Here's how the part is built. I have some questions about the finished solid (model axes, mm). Face numbers are marked on the shaded views. Coordinates: 2 decimals unless noted, no trailing zeros. Write each loop counter-clockwise with the first axis right and the second up, starting at its lowest first coordinate (ties: lowest second). Pieces come first, ordered by that corner, then holes.
Item 1: If I drill on line 1 (Z direction, x = 0, y = -9.75); line 2 (Z direction, x = 3, y = -16); line 3 (X direction, y = -3.5, z = -10), over which ranges is the centre line in solid material (lowest first)?
Item 2: I'm going to push flat-ended pins straight in: pin 1 Ø10 at (x, z) = (19, -15) entering from -Y; pin 2 Ø4 at (x, y) = (-11, -15.5) entering from +Z; pin 3 Ø8 at (x, y) = (10, -17) entering from +Z; pin 4 Ø6 at (x, z) = (6.5, -10.5) entering from +Y. Where does each tip first touch, or does it pass through?
Item 3: If we section it at D-D (y = -1.25): Please give me the cut outline in (x, z), then the cut area to 3 significant figures.
Item 4: We'd pull the mould along X, two halves only. Please class the marked faces 1, 2 and 3: +X half, -X half, draft (parallel to the pull), parting line (faces both ways), or undercut.
Item 5: If we section it at C-C (y = -8.75): Please give me the cut outline in (x, z).
from build123d import *

# Parameters (mm, degrees)
F0_R     = 24
F1_DEPTH = 3
F2_R     = 19
F3_DEPTH = 18
F5_D     = 36
F6_R     = 2.99999


# Not quite as in the source:
# - a fillet or chamfer is up to 0.001 mm smaller than in the source, because OpenCascade refuses the exact size


with BuildPart() as f1:
    # F0 (on Front) → F1 (new body)
    with BuildSketch(Plane.XZ):
        Circle(F0_R)
    extrude(amount=F1_DEPTH)

    # F2 (on face) → F3 (join)
    with BuildSketch(Plane.XZ.offset(3)):
        Circle(F2_R)
    extrude(amount=F3_DEPTH)

    # F5 (through all)
    with Locations(Plane(origin=(0, 0, 0), x_dir=(-1, 0, 0), z_dir=(0, 1, 0))):
        with Locations((0, 0)):
            Hole(F5_D / 2)

    # F6 (radius 3 in the source; OpenCascade refuses exactly that, so slightly less here)
    f6_edges = [f1.edges().sort_by_distance(p)[0] for p in [
        (-24, 0, 0),
        (18, 0, 0),
    ]]
    fillet(f6_edges, radius=F6_R)


solid = f1.part
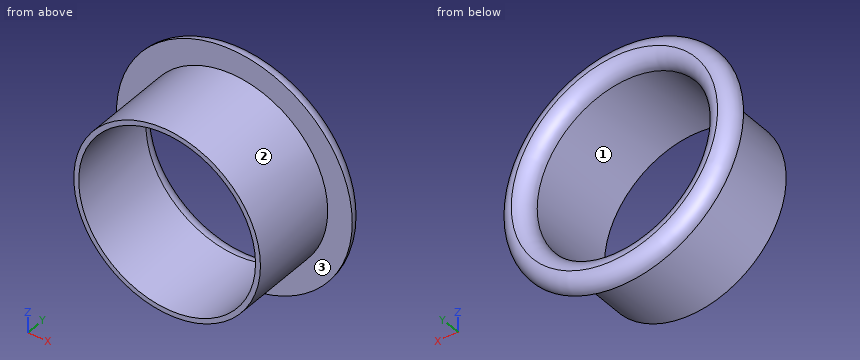
Answer list:
1. line 1: z = -19 to -18, 18 to 19
1. line 2: z = -18.76 to -17.75, 17.75 to 18.76
1. line 3: x = -16.16 to -14.97, 14.97 to 16.16
2. pin 1: stops at y = -3
2. pin 2: stops at z = 16.73
2. pin 3: stops at z = 18.03
2. pin 4: passes through
3. outline: circle Ø46.87 at (0, 0); hole circle Ø37.13 at (0, 0)
3. area: 643 mm2
4. face 1: undercut
4. face 2: parting line
4. face 3: draft
5. outline: circle Ø38 at (0, 0); hole circle Ø36 at (0, 0)
